```python
from build123d import *

# Parameters (mm, degrees)
SKETCH1_R               = 140
BOSS_EXTRUDE1_DEPTH     = 7.5
CUT_EXTRUDE1_DEPTH      = 199.557296517
CUT_EXTRUDE1_DEPTH_BACK = 199.557296517
SKETCH2_R               = 97.5
SKETCH3_R               = 105
BOSS_EXTRUDE2_DEPTH     = 45
SKETCH5_R               = 50
CUT_EXTRUDE2_DEPTH      = 207.881608656
SKETCH7_R               = 7.5
CUT_EXTRUDE3_DEPTH      = 207.881608656
CIRPATTERN1_COUNT       = 5
SKETCH9_W               = 15
SKETCH9_H               = 7
CUT_EXTRUDE4_DEPTH      = 318.421250076
CIRPATTERN2_COUNT       = 30
SKETCH11_R              = 96.873816077
CUT_EXTRUDE5_DEPTH      = 35
CUT_EXTRUDE6_START      = -35
SKETCH12_R              = 97.5
CUT_EXTRUDE6_DEPTH      = 35


with BuildPart() as part:
    # Sketch1 → Boss-Extrude1 (new, symmetric)
    with BuildSketch(Plane(origin=(0, 0, 0), x_dir=(1, 0, 0), z_dir=(0, 1, 0))):
        with Locations(Location((0, 0, 0), (0, 0, 270))):
            Circle(SKETCH1_R)
    extrude(amount=BOSS_EXTRUDE1_DEPTH, both=True)

    # Sketch2 → Cut-Extrude1 (cut, two sides: drawn at the far end of the back side and taken through both)
    with BuildSketch(Plane(origin=(0, 7.5, 0), x_dir=(1, 0, 0), z_dir=(0, 1, 0)).offset(-CUT_EXTRUDE1_DEPTH_BACK)):
        with Locations(Location((0, 0, 0), (0, 0, 270))):
            Circle(SKETCH2_R)
    extrude(amount=CUT_EXTRUDE1_DEPTH + CUT_EXTRUDE1_DEPTH_BACK, mode=Mode.SUBTRACT)

    # Sketch3 → Boss-Extrude2 (add)
    with BuildSketch(Plane(origin=(0, 7.5, 0), x_dir=(1, 0, 0), z_dir=(0, 1, 0))):
        with Locations(Location((0, 0, 0), (0, 0, 90))):
            Circle(SKETCH3_R)
    extrude(amount=BOSS_EXTRUDE2_DEPTH)

    # Sketch5 → Cut-Extrude2 (cut, through all)
    with BuildSketch(Plane(origin=(0, 52.5, 0), x_dir=(1, 0, 0), z_dir=(0, 1, 0))):
        with Locations(Location((0, 0, 0), (0, 0, 270))):
            Circle(SKETCH5_R)
    extrude(amount=-CUT_EXTRUDE2_DEPTH, mode=Mode.SUBTRACT)

    # Sketch7 → Cut-Extrude3 (cut, symmetric)
    with BuildSketch(Plane(origin=(0, 52.5, 0), x_dir=(1, 0, 0), z_dir=(0, 1, 0))):
        with Locations(Location((0, 80, 0), (0, 0, 270))):
            Circle(SKETCH7_R)
    cut_extrude3 = extrude(amount=CUT_EXTRUDE3_DEPTH, both=True, mode=Mode.SUBTRACT)

    # CirPattern1: Cut-Extrude3 ×5 about axis
    cirpattern1_axis = Axis((0, 0, 0), (0, 1, 0))
    for i in range(1, CIRPATTERN1_COUNT):
        add(cut_extrude3.rotate(cirpattern1_axis, i * 360 / CIRPATTERN1_COUNT), mode=Mode.SUBTRACT)

    # Sketch9 → Cut-Extrude4 (cut, symmetric)
    with BuildSketch(Plane(origin=(140, 0, 0), x_dir=(0, 0, -1), z_dir=(1, 0, 0))):
        Rectangle(SKETCH9_W, SKETCH9_H)
    cut_extrude4 = extrude(amount=CUT_EXTRUDE4_DEPTH, both=True, mode=Mode.SUBTRACT)

    # CirPattern2: Cut-Extrude4 ×30 about axis
    cirpattern2_axis = Axis((0, 0, 0), (0, 1, 0))
    for i in range(1, CIRPATTERN2_COUNT):
        add(cut_extrude4.rotate(cirpattern2_axis, i * 360 / CIRPATTERN2_COUNT), mode=Mode.SUBTRACT)

    # Sketch11 → Cut-Extrude5 (cut)
    with BuildSketch(Plane.XZ.offset(-7.5)):
        with Locations(Location((0, 0, 0), (0, 0, 270))):
            Circle(SKETCH11_R)
    extrude(amount=-CUT_EXTRUDE5_DEPTH, mode=Mode.SUBTRACT)

    # Sketch12 → Cut-Extrude6 (cut)
    with BuildSketch(Plane.XZ.offset(-7.5).offset(CUT_EXTRUDE6_START)):
        with Locations(Location((0, 0, 0), (0, 0, 90))):
            Circle(SKETCH12_R)
    extrude(amount=CUT_EXTRUDE6_DEPTH, mode=Mode.SUBTRACT)


solid = part.part
```
Could you check a few things on this model? Use its own coordinates, in mm. A direction names the side the tool comes from. Round coordinates to 2 decimals unless told otherwise and drop trailing zeros. Write each loop counter-clockwise with the first axis right and the second up, starting at its lowest first coordinate (ties: lowest second). Pieces come first, ordered by that corner, then holes. Notation, with made-up numbers: M 8,68.5 L 55,68.5 A20 cw 55,92.5 Z; hole C 5,70 d4. An arc over 180 degrees is marked long. Answer in a Markdown table with one row per item. Add a question column.
Q1. On a 3-axis mill with a long thin cutter (end or side, diameter ignored), from which of +Z, -Z, +X, -X, +Y, -Y can I reach the whole of each face in a straight line? I mean faces 3 (the flat face through (119, 3.5, 0)), 4 (the cylindrical face through (50.37, 47.57, 58.01)), 5 (the flat face through (-73.921, -0.049, -93.306)). Say none if no direction works.
Q2. Imagine slicing it at A-A (z = 0). Please give me the cut outline in (x, y), then the cut area to 4 significant figures.
Q3. Imagine slicing it at C-C (z = 40.5). Please give me the cut outline in (x, y).
Q4. Imagine slicing it at D-D (y = 39). Please give me the cut outline in (x, z), then the cut area to 3 significant figures.
Q5. Imagine slicing it at B-B (x = 112). Give the number of separate pieces and of enclosed holes in the cut face, then the cut area to 3 significant figures.
Q6. If I drill on line 1 (Y direction, x = 102.5, z = -39.5); line 2 (Z direction, x = 79, y = 0); line 3 (Y direction, x = -16.5, z = -47.5), over which ranges is the centre line in solid material (lowest first)? Write a range as from..to.
Q7. Will these pins go through, and if not, where does the flat tip stop? pin 1 Ø5 at (x, z) = (110, 30) entering from +Y; pin 2 Ø1.5 at (y, z) = (36, 71) entering from -X; pin 3 Ø7.5 at (x, y) = (-124.5, -0.5) entering from -Z.
Q8. If we mould it in two halves opening along X, with no side actions, what happens to faces 1 (the flat face through (-29, -7.5, -95)), 2 (the flat face through (37, -3.5, 112))? For each: +X half, -X half, draft (parallel to the pull), parting line (faces both ways), or undercut.
Values:
| question | item | result |
|---|---|---|
| 1 | face 3 | +X, -X |
| 1 | face 4 | +Y, -Y |
| 1 | face 5 | none |
| 2 | outline | M -140,-7.5 L -97.5,-7.5 L -97.5,-3.5 L -140,-3.5 Z; M -140,3.5 L -97.5,3.5 L -97.5,42.5 L -50,42.5 L -50,52.5 L -105,52.5 L -105,7.5 L -140,7.5 Z; M 50,42.5 L 97.5,42.5 L 97.5,3.5 L 140,3.5 L 140,7.5 L 105,7.5 L 105,52.5 L 50,52.5 Z; M 97.5,-7.5 L 140,-7.5 L 140,-3.5 L 97.5,-3.5 Z |
| 2 | area | 2,305 mm^2 |
| 3 | outline | M -134.01,-7.5 L -88.69,-7.5 L -88.69,-3.5 L -109.4,-3.5 L -109.4,3.5 L -88.69,3.5 L -88.69,42.5 L -29.32,42.5 L -29.32,52.5 L -96.87,52.5 L -96.87,7.5 L -134.01,7.5 Z; M 29.32,42.5 L 88.69,42.5 L 88.69,3.5 L 109.4,3.5 L 109.4,-3.5 L 88.69,-3.5 L 88.69,-7.5 L 134.01,-7.5 L 134.01,7.5 L 96.87,7.5 L 96.87,52.5 L 29.32,52.5 Z |
| 4 | outline | C 0,0 d210; hole C 0,0 d195 |
| 4 | area | 4,770 mm^2 |
| 5 | separate pieces | 1 |
| 5 | enclosed holes | 5 |
| 5 | area | 1,800 mm^2 |
| 6 | line 1 | -7.5..-3.5, 3.5..7.5 |
| 6 | line 2 | -115.58..-98.95, -76.53..-66.67, 66.67..76.53, 98.95..115.58 |
| 6 | line 3 | 42.5..52.5 |
| 7 | pin 1 | y = 7.5 |
| 7 | pin 2 | x = -78.04 |
| 7 | pin 3 | z = -70.85 |
| 8 | face 1 | draft |
| 8 | face 2 | undercut |
